Input: dimensioned drawing with shaded views. Units: mm. Origin: part minimum x, y, z. Round coordinates to 2 decimals unless told otherwise and drop trailing zeros. Loops run counter-clockwise (first coordinate to the right, second up) from the corner with the lowest first, then second, coordinate; pieces in that order, holes last. Notation, with made-up numbers: (77, 58.25) - (81, 58.25) arc R18 ccw to (81, 70.25) - close; hole circle Ø8 at (65.25, -8.5). An arc over 180 degrees is marked (long way). Answer as a JSON object with one key per item and string values. Group by question number.
Item 1: Line query: line 1 (X direction, y = 13.1, z = 7.5); line 2 (X direction, y = 2.8, z = 3.5); line 3 (Y direction, x = 3.75, z = 6.5). Output: solid intervals per line, ascending.
Item 2: Draft query along X for the marked faces 1, 2, 3 and 4. Return one class per face: released by +X, released by -X, zero draft, split by the parting line, or undercut.
Item 3: Section A-A (x = 2.8). Return the cut outline in (y, z).
Item 4: First-contact query: pin 1 (2.5 mm diameter, centred on x = 25, y = 13.1, fed in from -Z). Flat tip, straight axial feed; report the tip coordinate or a pass-through.
Item 5: Section C-C (z = 9.75). Return the cut outline in (x, y), plus the area to 3 significant figures.
Item 6: Section B-B (y = 13.1). Return the cut outline in (x, z).
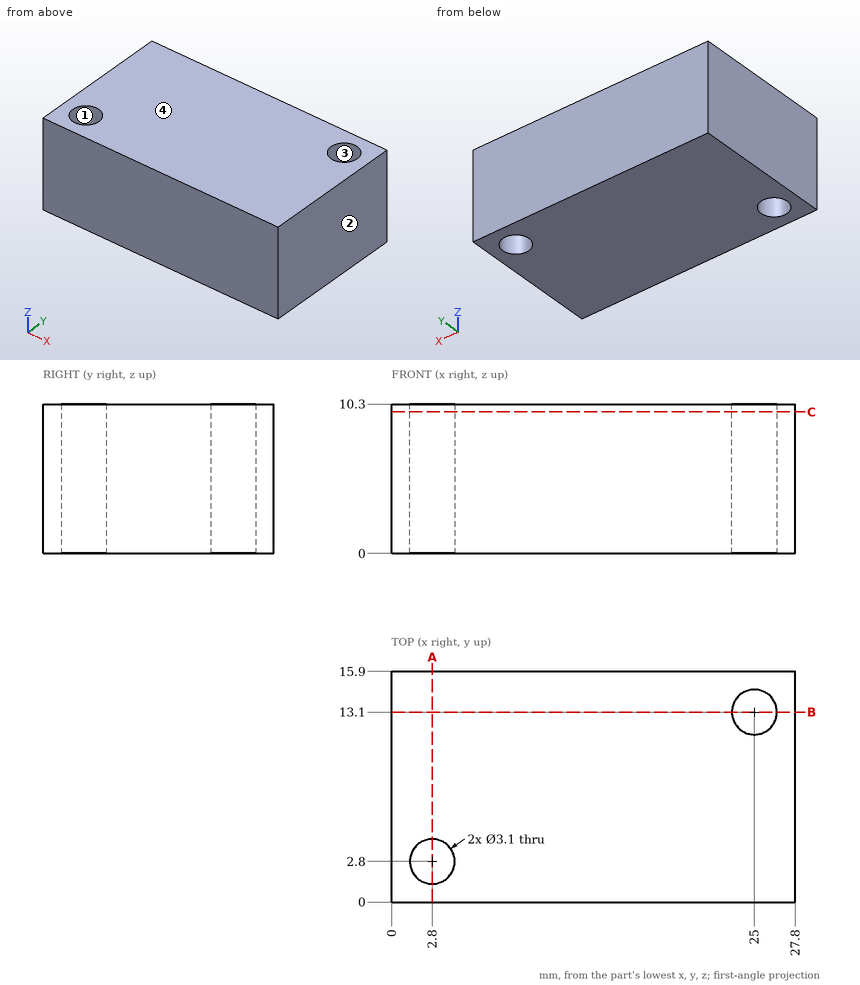
Values:
{
 "1": {"line 1": "x = 0 to 23.45, 26.55 to 27.8", "line 2": "x = 0 to 1.25, 4.35 to 27.8", "line 3": "y = 0 to 1.58, 4.02 to 15.9"},
 "2": {"face 1": "undercut", "face 2": "released by +X", "face 3": "undercut", "face 4": "zero draft"},
 "3": {"outline": "(0, 0) - (1.25, 0) - (1.25, 10.3) - (0, 10.3) - close; (4.35, 0) - (15.9, 0) - (15.9, 10.3) - (4.35, 10.3) - close"},
 "4": {"pin 1": "passes through"},
 "5": {"outline": "(0, 0) - (27.8, 0) - (27.8, 15.9) - (0, 15.9) - close; hole circle Ø3.1 at (2.8, 2.8); hole circle Ø3.1 at (25, 13.1)", "area": "427 mm^2"},
 "6": {"outline": "(0, 0) - (23.45, 0) - (23.45, 10.3) - (0, 10.3) - close; (26.55, 0) - (27.8, 0) - (27.8, 10.3) - (26.55, 10.3) - close"}
}
